```python
from build123d import *

# Parameters (mm, degrees)
F0_W     = 652
F0_H     = 829
F1_DEPTH = 2.5
F3_D     = 38
F4_SIZE  = 1


with BuildPart() as f1:
    # F0 (on Top) → F1 (new body, symmetric)
    with BuildSketch(Plane.XY):
        Rectangle(F0_W, F0_H)
    extrude(amount=F1_DEPTH, both=True)

    # F3 (through all)
    with Locations(Plane.XY.offset(2.5)):
        with Locations((-95, -271.5)):
            Hole(F3_D / 2)

    # F4
    f4_edges = [f1.edges().sort_by_distance(p)[0] for p in [
        (0, -414.5, -2.5),
        (-326, 0, -2.5),
        (0, 414.5, -2.5),
        (326, 0, -2.5),
        (326, 0, 2.5),
        (0, 414.5, 2.5),
        (-326, 0, 2.5),
        (0, -414.5, 2.5),
    ]]
    chamfer(f4_edges, length=F4_SIZE)


solid = f1.part
```
CAD build for the part. Positions are in the model's coordinates, mm. Give positions to 0.01 mm unless a question says otherwise; leave off trailing zeros. Order: outer loops, then holes, each group sorted by start corner. A loop starts at its lowest first (then second) coordinate and runs counter-clockwise, first axis right, second up.
(1) Drill centre lines: L1, parallel to Y at x = -95, z = 0.55; L2, parallel to Y at x = -99.5, z = 1.3; L3, parallel to X at y = -86, z = 1.95. Where is each one in solid material? Low to high.
(2) Saw through at B-B, the plane y = -271.5. Give the cut face in (x, z), then the cut area to 3 significant figures.
(3) Mould opens along X. For faces 1 (the cylindrical face through (-90.881, -290.048, -0.035)), 2 (the flat face through (-5, 6, -2.5)) say: released by +X, released by -X, zero draft, split by the parting line, or undercut.
(4) Saw through at A-A, the plane x = -95. Give the cut face in (y, z).
Results found:
1. L1: y = -414.5 to -290.5, -252.5 to 414.5
1. L2: y = -414.5 to -289.96, -253.04 to 414.5
1. L3: x = -325.55 to 325.55
2. outline: (-326, -1.5) - (-325, -2.5) - (-114, -2.5) - (-114, 2.5) - (-325, 2.5) - (-326, 1.5) - close; (-76, -2.5) - (325, -2.5) - (326, -1.5) - (326, 1.5) - (325, 2.5) - (-76, 2.5) - close
2. area: 3,070 mm2
3. face 1: undercut
3. face 2: zero draft
4. outline: (-414.5, -1.5) - (-413.5, -2.5) - (-290.5, -2.5) - (-290.5, 2.5) - (-413.5, 2.5) - (-414.5, 1.5) - close; (-252.5, -2.5) - (413.5, -2.5) - (414.5, -1.5) - (414.5, 1.5) - (413.5, 2.5) - (-252.5, 2.5) - close
